```python
from build123d import *

# Parameters (mm, degrees)
F_1_4_INCH_THICKNESS_DEPTH = 3.175
FILLET1_R                  = 76.2


with BuildPart() as part:
    # Sketch1 → 1/4 Inch Thickness (new, symmetric)
    with BuildSketch(Plane.XY):
        Polygon((-63.5, 6.35), (63.5, 6.35), (63.5, 12.7), (101.6, 12.7), (101.6, -12.7), (63.5, -12.7), (63.5, -6.35), (-63.5, -6.35), (-63.5, -12.7), (-101.6, -12.7), (-101.6, 12.7), (-63.5, 12.7), align=None)
    extrude(amount=F_1_4_INCH_THICKNESS_DEPTH, both=True)

    # Fillet1
    # the kernel refuses this fillet: 76.2 mm, written as the material it adds along each edge
    with BuildSketch(Plane(origin=(63.5, -6.35, 3.175), x_dir=(-1, 0, 0), z_dir=(0, 0, -1))) as fillet1_piece_1:
        with BuildLine():
            CenterArc((30.453530173, -76.2), FILLET1_R, 90, 23.556464309)
            Line((0, -6.35), (-0.609070603, -4.953))
            ThreePointArc((-0.609070603, -4.953), (-1.524, -3.175), (-1.524, 0))
            Line((-1.524, 0), (0, 1.524))
            Line((0, 1.524), (30.453530173, 1.524))
            Line((30.453530173, 1.524), (30.453530173, 0))
        make_face()
    extrude(amount=6.35)
    with BuildSketch(Plane(origin=(63.5, 6.35, 3.175), x_dir=(-1, 0, 0), z_dir=(0, 0, -1)), Plane(origin=(-63.5, 6.35, -3.175), x_dir=(1, 0, 0), z_dir=(0, 0, 1))) as fillet1_piece_2:
        with BuildLine():
            CenterArc((30.453530173, 76.2), FILLET1_R, 246.443535691, 23.556464309)
            Line((0, 6.35), (-0.609070603, 4.953))
            ThreePointArc((-0.609070603, 4.953), (-1.524, 3.175), (-1.524, 0))
            Line((-1.524, 0), (0, -1.524))
            Line((0, -1.524), (30.453530173, -1.524))
            Line((30.453530173, -1.524), (30.453530173, 0))
        make_face()
    extrude(amount=6.35)
    with BuildSketch(Plane(origin=(-63.5, -6.35, 3.175), x_dir=(0, -1, 0), z_dir=(0, 0, -1))) as fillet1_piece_3:
        with BuildLine():
            CenterArc((76.2, -30.453530173), FILLET1_R, 156.443535691, 23.556464309)
            Line((0, -30.453530173), (-1.524, -30.453530173))
            Line((-1.524, -30.453530173), (-1.524, 0))
            Line((-1.524, 0), (0, 1.524))
            ThreePointArc((0, 1.524), (3.175, 1.524), (4.953, 0.609070603))
            Line((4.953, 0.609070603), (6.35, 0))
        make_face()
    extrude(amount=6.35)


solid = part.part
```
Verification items for the finished model (mm, model axes). A direction names the side the tool comes from. Coordinates: 2 decimals unless noted, no trailing zeros. Order: outer loops, then holes, each group sorted by start corner. A loop starts at its lowest first (then second) coordinate and runs counter-clockwise, first axis right, second up. Notation, with made-up numbers: (71.25, -39.5) -> (113.25, -39.5) arc R7 ccw to (113.25, -35.5) -> close; hole circle Ø2 at (56, 53.25). An arc over 180 degrees is marked (long way). Answer as CSV lines item,"result". Start each with the question number.
1) Release check for a two-part mould opening along X. For faces 1 (the face through (-101.6, 0, 0)), 2 (the face through (-48.82, 8, -0.04)), 3 (the face through (83, -12.7, 0)) record: released by +X, released by -X, zero draft, split by the parting line, or undercut.
2) Cross-section at C-C, the plane x = -15. Record the boundary of the cut face in (y, z) (3 decimals).
3) Material ranges on L1, parallel to Y at x = -33.5, z = -1.5; L2, parallel to Y at x = 41, z = 2.5, recorded low to high. Write a range as [from, to].
4) Cross-section at B-B, the plane y = -11. Record the boundary of the cut face in (x, z) (3 decimals), then the cut area to 3 significant figures.
5) Cross-section at D-D, the plane x = 44. Record the boundary of the cut face in (y, z) (3 decimals).
6) Gauge pin test, flat end, axial feed: pin 1 Ø3 at (x, z) = (-16, -1.5) entering from +Y. Record the tip position at first contact, or that the pin passes through.
7) Cross-section at A-A, the plane z = 1.75. Record the boundary of the cut face in (x, y), then the cut area to 3 significant figures.
8) Set-up check for faces 4 (the face through (48.39, -7.91, 0.04)), 5 (the face through (48.82, 8, 0.04)), 6 (the face through (-1, 0, -3.175)): record each of +Z, -Z, +X, -X, +Y, -Y from which the full face is reachable in a straight line by a thin tool's end or side.
Conclusion:
1,face 1,"released by -X"
1,face 2,"undercut"
1,face 3,"zero draft"
2,outline,"(-6.35, -3.175) -> (6.35, -3.175) -> (6.35, 3.175) -> (-6.35, 3.175) -> close"
3,L1,"y = [-6.35, 6.35]"
3,L2,"y = [-6.77, 6.77]"
4,outline,"(-101.6, -3.175) -> (-59.258, -3.175) -> (-59.258, 3.175) -> (-101.6, 3.175) -> close; (59.258, -3.175) -> (101.6, -3.175) -> (101.6, 3.175) -> (59.258, 3.175) -> close"
4,area,"538 mm²"
5,outline,"(-7.141, -3.175) -> (7.141, -3.175) -> (7.141, 3.175) -> (-7.141, 3.175) -> close"
6,pin 1,"stops at y = 6.35"
7,outline,"(-101.6, -12.7) -> (-63.5, -12.7) arc R76.2 cw to (-33.05, -6.35) -> (33.05, -6.35) arc R76.2 cw to (63.5, -12.7) -> (101.6, -12.7) -> (101.6, 12.7) -> (63.5, 12.7) arc R76.2 cw to (33.05, 6.35) -> (-33.05, 6.35) arc R76.2 cw to (-63.5, 12.7) -> (-101.6, 12.7) -> close"
7,area,"3,800 mm²"
8,face 4,"+Z, -Z, -Y"
8,face 5,"+Z, -Z, +Y"
8,face 6,"-Z, +X, -X, +Y, -Y"
